```python
from build123d import *

# Parameters (mm, degrees)
IZIM1_R                                      = 5
IZIM1_R_2                                    = 4
Y_KSEKLIK_EKSTR_ZYON1_DEPTH                  = 4
IZIM2_R                                      = 1.5
Y_KSEKLIK_EKSTR_ZYON2_DEPTH                  = 60
Y_KSEKLIK_EKSTR_ZYON2_DIRECTION_2_REACH      = 13.874
Y_KSEKLIK_EKSTR_ZYON2_DIRECTION_2_END_RADIUS = 5
IZIM3_R                                      = 2.5
Y_KSEKLIK_EKSTR_ZYON3_DEPTH                  = 2


with BuildPart() as part:
    # Çizim1 → Yükseklik-Ekstrüzyon1 (new body)
    with BuildSketch(Plane.XY):
        Circle(IZIM1_R)
        Circle(IZIM1_R_2, mode=Mode.SUBTRACT)
    extrude(amount=Y_KSEKLIK_EKSTR_ZYON1_DEPTH)


with BuildPart() as y_kseklik_ekstr_zyon2_tool:
    # Çizim2 → Yükseklik-Ekstrüzyon2 (new body)
    with BuildSketch(Plane(origin=(5, 0, 0), x_dir=(0, 0, -1), z_dir=(1, 0, 0))):
        with Locations((-2, 0)):
            Circle(IZIM2_R)
    extrude(amount=Y_KSEKLIK_EKSTR_ZYON2_DEPTH)


with BuildPart() as part_1:
    add(part.part)


with BuildPart() as part_2:
    # Yükseklik-Ekstrüzyon2: joined with y_kseklik_ekstr_zyon2_tool
    add(part_1.part.fuse(y_kseklik_ekstr_zyon2_tool.part, tol=0.00001))

    # Yükseklik-Ekstrüzyon2 direction 2: up to this cylinder (the profile starts outside it)
    y_kseklik_ekstr_zyon2_direction_2_end = Plane(origin=(0, 0, 2), z_dir=(0, 0, -1)) * Cylinder(Y_KSEKLIK_EKSTR_ZYON2_DIRECTION_2_END_RADIUS, 38.748, mode=Mode.PRIVATE)
    # Çizim2 → Yükseklik-Ekstrüzyon2 direction 2 (add, up to the surface)
    with BuildSketch(Plane(origin=(5, 0, 0), x_dir=(0, 0, -1), z_dir=(1, 0, 0)), mode=Mode.PRIVATE) as y_kseklik_ekstr_zyon2_direction_2_sk1:
        with Locations((-2, 0)):
            Circle(IZIM2_R)
    y_kseklik_ekstr_zyon2_direction_2_tool1 = extrude(y_kseklik_ekstr_zyon2_direction_2_sk1.sketch, amount=-Y_KSEKLIK_EKSTR_ZYON2_DIRECTION_2_REACH, mode=Mode.PRIVATE) - y_kseklik_ekstr_zyon2_direction_2_end
    add(y_kseklik_ekstr_zyon2_direction_2_tool1.solids().sort_by_distance((5, 0, 2))[0])
    add(y_kseklik_ekstr_zyon2_direction_2_tool1.solids().sort_by_distance((5, 0, 2))[1])

    # Çizim3 → Yükseklik-Ekstrüzyon3 (add)
    with BuildSketch(Plane(origin=(65, 0, 0), x_dir=(0, 0, -1), z_dir=(1, 0, 0))):
        with Locations((-2, 0)):
            Circle(IZIM3_R)
    extrude(amount=Y_KSEKLIK_EKSTR_ZYON3_DEPTH)


solid = part_2.part
```
Design review of the part built by this model. Coordinates are the model's own, in mm. A direction names the side the tool comes from. Give positions to 0.01 mm unless a question says otherwise; leave off trailing zeros. Write each loop counter-clockwise with the first axis right and the second up, starting at its lowest first coordinate (ties: lowest second). Pieces come first, ordered by that corner, then holes.
(1) Clearance check with flat-ended pins moving along their axes: pin 1 Ø1 at (x, z) = (41, 3.5) entering from -Y; pin 2 Ø1.5 at (y, z) = (2, 3.5) entering from -X; pin 3 Ø1.5 at (y, z) = (-3.5, 1.5) entering from -X. State where each tip first meets the part, or that it passes through.
Checked values:
pin 1: stops at y = -1.12
pin 2: stops at x = -4.84
pin 3: stops at x = -4.18
(2) Add section A-A (x = 0). Give the boundary of the cut face in (y, z), and give its area (3 significant figures).
Checked values:
outline: (-5, 0) - (-4, 0) - (-4, 4) - (-5, 4) - close; (4, 0) - (5, 0) - (5, 4) - (4, 4) - close
area: 8.00 mm2
(3) Wall thickness on line 1 along Y through (x, z) = (0, 1.05); line 2 along X through (y, z) = (2, 2.65); line 3 along X through (y, z) = (2.25, 1.95): over which ranges is each line inside the solid? List them lowest first.
Checked values:
line 1: y = -5 to -4, 4 to 5
line 2: x = -4.58 to -3.46, 3.46 to 4.58, 65 to 67
line 3: x = -4.47 to -3.31, 3.31 to 4.47, 65 to 67
(4) Tool access review of faces 1 (the face through (-0.867, -3.905, 1.972)), 2 (the face through (65, -2, 2)): name each direction out of +Z, -Z, +X, -X, +Y, -Y from which nothing blocks a thin tool from reaching the whole face with its end or side.
Checked values:
face 1: +Z, -Z
face 2: none
(5) Mouldability with a two-part tool opening along X and no side actions: class faces 3 (the face through (67, 0, 2)), 4 (the face through (66, 0.1, 4.5)), 5 (the face through (34.46, 0.45, 0.57)) as +X half, -X half, draft (parallel to the pull), parting line (faces both ways), or undercut.
Checked values:
face 3: +X half
face 4: draft
face 5: undercut
(6) Add section B-B (z = 2). Give the boundary of the cut face in (x, y).
Checked values:
outline: (4.77, -1.5) - (65, -1.5) - (65, -2.5) - (67, -2.5) - (67, 2.5) - (65, 2.5) - (65, 1.5) - (4.77, 1.5) arc R5 ccw (long way) to start; hole circle Ø8 at (0, 0)
(7) Add section C-C (x = 47). Give the boundary of the cut face in (y, z), and give its area (3 significant figures).
Checked values:
outline: circle Ø3 at (0, 2)
area: 7.07 mm2
